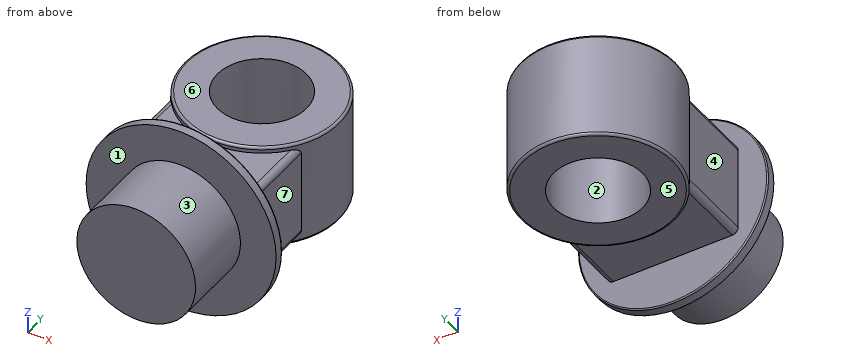
```python
from build123d import *

# Parameters (mm, degrees)
SKETCH1_R                = 100
BOSS_EXTRUDE1_DEPTH      = 120
SKETCH2_R                = 160
BOSS_EXTRUDE2_DEPTH      = 16
SKETCH3_R                = 130
SKETCH3_R_2              = 75
BOSS_EXTRUDE3_DEPTH      = 90
BOSS_EXTRUDE4_REACH      = 402.125
BOSS_EXTRUDE4_END_RADIUS = 130
SKETCH4_W                = 220
SKETCH4_H                = 160
FILLET1_R                = 2
FILLET2_R                = 4
FILLET3_R                = 10


with BuildPart() as part:
    # Sketch1 → Boss-Extrude1 (new body)
    with BuildSketch(Plane(origin=(0, 0, 0), x_dir=(1, 0, 0), z_dir=(0, 1, 0))):
        with Locations(Location((0, 0, 0), (0, 0, 270))):
            Circle(SKETCH1_R)
    extrude(amount=BOSS_EXTRUDE1_DEPTH)

    # Sketch2 → Boss-Extrude2 (add)
    with BuildSketch(Plane(origin=(0, 120, 0), x_dir=(1, 0, 0), z_dir=(0, 1, 0))):
        with Locations(Location((0, 0, 0), (0, 0, 270))):
            Circle(SKETCH2_R)
    extrude(amount=BOSS_EXTRUDE2_DEPTH)



with BuildPart() as body_2:
    # Sketch3 → Boss-Extrude3 (new, symmetric)
    with BuildSketch(Plane.XY):
        with Locations(Location((0, 336, 0), (0, 0, 180))):
            Circle(SKETCH3_R)
        with Locations(Location((0, 336, 0), (0, 0, 180))):
            Circle(SKETCH3_R_2, mode=Mode.SUBTRACT)
    extrude(amount=BOSS_EXTRUDE3_DEPTH, both=True)


with BuildPart() as part_1:
    add(part.part)

    add(body_2.part)  # Boss-Extrude4 merges body 2
    # Boss-Extrude4: up to this cylinder (the profile starts outside it)
    boss_extrude4_end = Plane(origin=(0, 336, 0), z_dir=(0, 0, -1)) * Cylinder(BOSS_EXTRUDE4_END_RADIUS, 1065.25, mode=Mode.PRIVATE)
    # Sketch4 → Boss-Extrude4 (add, up to the surface)
    with BuildSketch(Plane(origin=(0, 136, 0), x_dir=(1, 0, 0), z_dir=(0, 1, 0)), mode=Mode.PRIVATE) as boss_extrude4_sk1:
        Rectangle(SKETCH4_W, SKETCH4_H)
    boss_extrude4_tool1 = extrude(boss_extrude4_sk1.sketch, amount=BOSS_EXTRUDE4_REACH, mode=Mode.PRIVATE) - boss_extrude4_end
    add(boss_extrude4_tool1.solids().sort_by_distance((0, 136, 0))[0])

    # Fillet1
    fillet1_edges = [part_1.edges().sort_by_distance(p)[0] for p in [
        (0, 136, -160),
    ]]
    fillet(fillet1_edges, radius=FILLET1_R)

    # Fillet2
    fillet2_edges = [part_1.edges().sort_by_distance(p)[0] for p in [
        (130, 336, -90),
        (130, 336, 90),
    ]]
    fillet(fillet2_edges, radius=FILLET2_R)

    # Fillet3
    fillet3_edges = [part_1.edges().sort_by_distance(p)[0] for p in [
        (-110, 201.358983849, 80),
        (-110, 201.358983849, -80),
        (110, 201.358983849, 80),
        (110, 201.358983849, -80),
    ]]
    fillet(fillet3_edges, radius=FILLET3_R)


solid = part_1.part
```
Part model, mm, in its own coordinate system. Face numbers are marked on the shaded views. A direction names the side the tool comes from. Give positions to 0.01 mm unless a question says otherwise; leave off trailing zeros. Write each loop counter-clockwise with the first axis right and the second up, starting at its lowest first coordinate (ties: lowest second). Pieces come first, ordered by that corner, then holes. Notation, with made-up numbers: (70.5, -15) -> (88.5, -15) arc R27 ccw to (88.5, 5) -> close; hole circle Ø2 at (-15, 46). An arc over 180 degrees is marked (long way). Put each result on its own line as item: value. Start each with the question number.
Item 1: Wall check: L1, parallel to Y at x = 0, z = 10; L2, parallel to X at y = 336, z = -35; L3, parallel to Y at x = -74, z = -100. Give the ranges that are in metal, low to high. Write a range as [from, to].
Item 2: Which spindle directions (+Z, -Z, +X, -X, +Y, -Y) get a long thin tool onto all of the face, cutting with end or side? Do the marked faces 4, 5, 6 and 7. Say none if no direction does.
Item 3: Cut at B-B (z = 0). List the corners of the cut face in (x, y), then the cut area to 3 significant figures.
Item 4: Cut at A-A (y = 336). List the corners of the cut face in (x, z).
Item 5: Pin check, flat tips, straight feed: pin 1 Ø4 at (x, y) = (-67.5, 383.5) entering from -Z; pin 2 Ø4 at (y, z) = (111.5, -85.5) entering from +X (3 decimals); pin 3 Ø1 at (x, y) = (-114.5, 363) entering from +Z. Stop position of each tip, or through.
Item 6: Cut at D-D (y = 161). List the corners of the cut face in (x, z).
Item 7: Pull direction Y, two halves, no side cores. Call the marked faces 1, 2 and 3: pulls with the +Y half, pulls with the -Y half, needs draft (parallel to the pull), parting line crosses it, or undercut.
Item 8: Cut at C-C (x = 0). List the corners of the cut face in (y, z).
Answer list:
1. L1: y = [0, 261], [411, 466]
1. L2: x = [-130, -75], [75, 130]
1. L3: y = [120, 136]
2. face 4: +Z, -Z, -X
2. face 5: -Z, +X, -X, +Y
2. face 6: +Z, +X, -X, +Y
2. face 7: +Z, -Z, +X
3. outline: (-160, 120) -> (-100, 120) -> (-100, 0) -> (100, 0) -> (100, 120) -> (160, 120) -> (160, 134) arc R2 ccw to (158, 136) -> (110, 136) -> (110, 266.72) arc R130 ccw (long way) to (-110, 266.72) -> (-110, 136) -> (-158, 136) arc R2 ccw to (-160, 134) -> close; hole circle Ø150 at (0, 336)
3. area: 83,900 mm2
4. outline: (-130, -86) arc R4 ccw to (-126, -90) -> (-75, -90) -> (-75, 90) -> (-126, 90) arc R4 ccw to (-130, 86) -> close; (75, -90) -> (126, -90) arc R4 ccw to (130, -86) -> (130, 86) arc R4 ccw to (126, 90) -> (75, 90) -> close
5. pin 1: stops at z = -90
5. pin 2: stops at x = 55.025
5. pin 3: stops at z = 90
6. outline: (-110, -70) arc R10 ccw to (-100, -80) -> (100, -80) arc R10 ccw to (110, -70) -> (110, 70) arc R10 ccw to (100, 80) -> (-100, 80) arc R10 ccw to (-110, 70) -> close
7. face 1: pulls with the -Y half
7. face 2: undercut
7. face 3: needs draft
8. outline: (0, -100) -> (120, -100) -> (120, -160) -> (134, -160) arc R2 ccw to (136, -158) -> (136, -80) -> (206, -80) -> (206, -86) arc R4 ccw to (210, -90) -> (261, -90) -> (261, 90) -> (210, 90) arc R4 ccw to (206, 86) -> (206, 80) -> (136, 80) -> (136, 158) arc R2 ccw to (134, 160) -> (120, 160) -> (120, 100) -> (0, 100) -> close; (411, -90) -> (462, -90) arc R4 ccw to (466, -86) -> (466, 86) arc R4 ccw to (462, 90) -> (411, 90) -> close
